from build123d import *

# Parameters (mm, degrees)
F1_DEPTH = 12.7


with BuildPart() as f1:
    # F0 (on Top) → F1 (new body)
    with BuildSketch(Plane.XY):
        Polygon((0, -15.680935), (0, 29.021675), (-3.516382, 29.021675), (-5.095464, 32.706197), (-7.034861, 23.75273), (-51.050033, 32.706197), (-65.449044, 0), (-59.080428, 2.729409), (-38.705469, -1.482393), (-36.721308, -5.629899), (-31.266223, -3.020194), (-8.013232, -7.826927), align=None)
        Polygon((3.516382, 29.021675), (0, 29.021675), (0, -15.680935), (8.013232, -7.826927), (31.266223, -3.020194), (36.721308, -5.629899), (38.705469, -1.482393), (59.080428, 2.729409), (65.449044, 0), (51.050033, 32.706197), (7.034861, 23.75273), (5.095464, 32.706197), align=None)
    extrude(amount=F1_DEPTH)


solid = f1.part
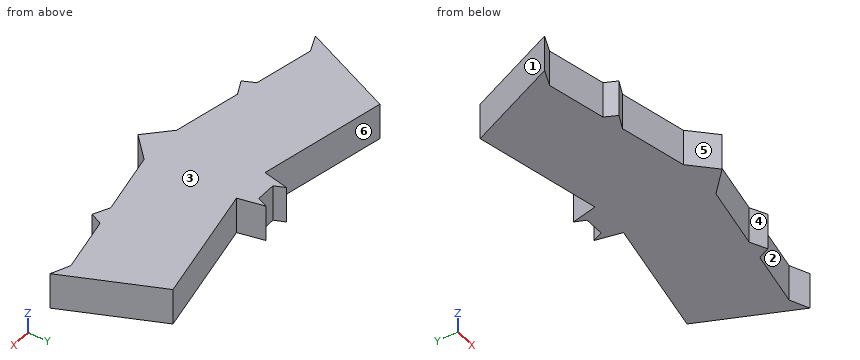
The model under review builds one solid part; all positions refer to its coordinate system, in mm. Face numbers are marked on the shaded views. A direction names the side the tool comes from. Round coordinates to 2 decimals unless told otherwise and drop trailing zeros. Order: outer loops, then holes, each group sorted by start corner. A loop starts at its lowest first (then second) coordinate and runs counter-clockwise, first axis right, second up. Notation, with made-up numbers: (1.5, 22) -> (59.5, 22) arc R23 cw to (59.5, 36) -> close; hole circle Ø2 at (-13, -22.5). An arc over 180 degrees is marked (long way). Return JSON: item names as keys, results as strings.
1. The part is to be moulded in two halves that separate along X. For the marked faces 1, 2 and 3, say which applies: +X half, -X half, draft (parallel to the pull), parting line (faces both ways), or undercut.
Answer block:
{"face 1": "-X half", "face 2": "undercut", "face 3": "draft"}
2. For L1, parallel to Y at x = -20, z = 1; L2, parallel to X at y = 15, z = 2.75; L3, parallel to Y at x = -41, z = 7.5, list the stretches that pass through material, from the lowest coordinate up. Write a range as [from, to].
Answer block:
{"L1": "y = [-5.35, 26.39]", "L2": "x = [-58.85, 58.85]", "L3": "y = [-1.01, 30.66]"}
3. Take a section at C-C (x = -20.5). Write out the cut boundary in (y, z).
Answer block:
{"outline": "(-5.25, 0) -> (26.49, 0) -> (26.49, 12.7) -> (-5.25, 12.7) -> close"}
4. Insertion check: P1, Ø3, axis at y = 16, z = 10.5, coming from the +X side; P2, Ø1, axis at x = 31.5, z = 5, coming from the +Y side; P3, Ø5, axis at y = 8, z = 2.5, coming from the -X side. Each pin has a flat end and moves straight along its axis. Give the tip position at first contact, or say it passes through.
Answer block:
{"P1": "stops at x = 59.07", "P2": "stops at y = 28.83", "P3": "stops at x = -63.03"}
5. Take a section at A-A (y = 25). Write out the cut boundary in (x, z), then the cut area to 3 significant figures.
Answer block:
{"outline": "(-54.44, 0) -> (-13.17, 0) -> (-13.17, 12.7) -> (-54.44, 12.7) -> close; (-6.76, 0) -> (6.76, 0) -> (6.76, 12.7) -> (-6.76, 12.7) -> close; (13.17, 0) -> (54.44, 0) -> (54.44, 12.7) -> (13.17, 12.7) -> close", "area": "1,220 mm²"}
6. Take a section at B-B (z = 5.5). Write out the cut boundary in (x, y), then the cut area to 3 significant figures.
Answer block:
{"outline": "(-65.45, 0) -> (-59.08, 2.73) -> (-38.71, -1.48) -> (-36.72, -5.63) -> (-31.27, -3.02) -> (-8.01, -7.83) -> (0, -15.68) -> (8.01, -7.83) -> (31.27, -3.02) -> (36.72, -5.63) -> (38.71, -1.48) -> (59.08, 2.73) -> (65.45, 0) -> (51.05, 32.71) -> (7.03, 23.75) -> (5.1, 32.71) -> (3.52, 29.02) -> (-3.52, 29.02) -> (-5.1, 32.71) -> (-7.03, 23.75) -> (-51.05, 32.71) -> close", "area": "3,830 mm²"}
7. For the marked faces 4, 5 and 6, list the 3-axis set-ups (+Z, -Z, +X, -X, +Y, -Y) from which the entire face can be reached by the end or side of a thin tool; tool diameter is ignored.
Answer block:
{"face 4": "+Z, -Z, -Y", "face 5": "+Z, -Z, -X, -Y", "face 6": "+Z, -Z, +Y"}
8. Take a section at D-D (y = 17). Write out the cut boundary in (x, z), then the cut area to 3 significant figures.
Answer block:
{"outline": "(-57.96, 0) -> (57.96, 0) -> (57.96, 12.7) -> (-57.96, 12.7) -> close", "area": "1,470 mm²"}
